Read the model definition and answer for the solid it produces. Units are mm, in the model's axes. A direction names the side the tool comes from. Coordinates: 2 decimals unless noted, no trailing zeros. Loops run counter-clockwise (first coordinate to the right, second up) from the corner with the lowest first, then second, coordinate; pieces in that order, holes last. Notation, with made-up numbers: (64, -11) - (98, -11) arc R28 cw to (98, 21) - close; hole circle Ø8 at (41.5, 37.5). An arc over 180 degrees is marked (long way). Use one line per item in the form item = value.
from build123d import *

# Parameters (mm, degrees)
F0_W      = 100
F0_H      = 100
F1_DEPTH  = 100
F2_R      = 5
F3_DEPTH  = 100
F5_DEPTH  = 25
F8_DEPTH  = 25
F10_DEPTH = 25
F11_DEPTH = 25
F12_SIZE  = 5
F14_DEPTH = 10


with BuildPart() as f1:
    # F0 (on Top) → F1 (new body)
    with BuildSketch(Plane.XY):
        with Locations((50, 50)):
            Rectangle(F0_W, F0_H)
    extrude(amount=F1_DEPTH)

    # F2 (on face) → F3 (cut)
    with BuildSketch(Plane.XY.offset(100)):
        with Locations((15, 25)):
            Circle(F2_R)
        with Locations((15, 50)):
            Circle(F2_R)
        with Locations((15, 75)):
            Circle(F2_R)
    extrude(amount=-F3_DEPTH, mode=Mode.SUBTRACT)

    # F4 (on face) → F5 (cut)
    with BuildSketch(Plane.XZ):
        with BuildLine():
            Line((39.7404471785, 30), (50, 30))
            Line((50, 30), (100, 30))
            Line((100, 30), (100, 100))
            Line((100, 100), (29.7404471785, 100))
            Line((29.7404471785, 100), (29.7404471785, 40))
            ThreePointArc((29.7404471785, 40), (32.6693793666, 32.9289321881), (39.7404471785, 30))
        make_face()
    extrude(amount=-F5_DEPTH, mode=Mode.SUBTRACT)

    # F7 (on face) → F8 (cut)
    with BuildSketch(Plane(origin=(0, 100, 0), x_dir=(-1, 0, 0), z_dir=(0, 1, 0))):
        with BuildLine():
            Line((-100, 30), (-39.7373309731, 30))
            ThreePointArc((-39.7373309731, 30), (-32.6662631613, 32.9289321881), (-29.7373309731, 40))
            Line((-29.7373309731, 40), (-29.7373309731, 100))
            Line((-29.7373309731, 100), (-100, 100))
            Line((-100, 100), (-100, 30))
        make_face()
    extrude(amount=-F8_DEPTH, mode=Mode.SUBTRACT)

    # F9 (on face) → F10 (cut)
    with BuildSketch(Plane.XZ.offset(-25)):
        Polygon((100, 100), (29.7404471785, 100), (100, 30), align=None)
    extrude(amount=-F10_DEPTH, mode=Mode.SUBTRACT)

    # F11 (cut): a face of the model
    f11_faces = [f1.faces().sort_by_distance(p)[0] for p in [
        (76.5801490595, 50, 76.6666666667),
    ]]
    extrude(f11_faces, amount=-F11_DEPTH, mode=Mode.SUBTRACT)

    # F12
    f12_edges = [f1.edges().sort_by_distance(p)[0] for p in [
        (100, 0, 15),
        (100, 100, 15),
    ]]
    chamfer(f12_edges, length=F12_SIZE)

    # F13 (on face) → F14 (cut)
    with BuildSketch(Plane.YZ.offset(100)):
        Polygon((39.8671727255, 10), (49.8671727255, 10), (59.8671727255, 10), (59.8671727255, 20.3688494319), (39.8671727255, 20.3688494319), align=None)
    extrude(amount=-F14_DEPTH, mode=Mode.SUBTRACT)


solid = f1.part
Item 1: The part is cut by section B-B on y = 50. Give the vertices of the cut face in (x, z), plus the area to 3 significant figures.
Results below:
outline = (0, 0) - (10, 0) - (10, 100) - (0, 100) - close; (20, 0) - (100, 0) - (100, 10) - (90, 10) - (90, 20.37) - (100, 20.37) - (100, 30) - (29.74, 100) - (20, 100) - close
area = 6,440 mm²
Item 2: Each of these flat-tipped pins is pushed along its axis until it touches: P1, Ø7.5, axis at y = 13.5, z = 69.5, coming from the +X side; P2, Ø20, axis at x = 56, y = 89, coming from the +Z side; P3, Ø3, axis at x = 97, z = 15.5, coming from the +Y side; P4, Ø6, axis at x = 15, y = 25, coming from the -Z side. Where does it stop, or does it pass through?
Results below:
P1 = 29.74
P2 = 30
P3 = 99.5
P4 = through
Item 3: The part is cut by section A-A on x = 15. Give the vertices of the cut face in (y, z).
Results below:
outline = (0, 0) - (20, 0) - (20, 100) - (0, 100) - close; (30, 0) - (45, 0) - (45, 100) - (30, 100) - close; (55, 0) - (70, 0) - (70, 100) - (55, 100) - close; (80, 0) - (100, 0) - (100, 100) - (80, 100) - close
Item 4: The part is cut by section C-C on z = 8.5. Give the vertices of the cut face in (x, y), plus the area to 3 significant figures.
Results below:
outline = (0, 0) - (95, 0) - (100, 5) - (100, 95) - (95, 100) - (0, 100) - close; hole circle Ø10 at (15, 25); hole circle Ø10 at (15, 50); hole circle Ø10 at (15, 75)
area = 9,740 mm²
Item 5: Which of the six approach directions +Z, -Z, +X, -X, +Y, -Y give full straight-line access (tool end or side, diameter ignored) to faces 4 (the flat face through (69, 12, 30)), 5 (the flat face through (97, 2, 15)), 6 (the flat face through (95, 50, 20.369)), 7 (the flat face through (29.737, 88, 70))?
Results below:
face_4 = +Z, +X, -Y
face_5 = +Z, -Z, +X, -Y
face_6 = +X
face_7 = +Z, +X, +Y
Item 6: The part is cut by section D-D on y = 86. Give the vertices of the cut face in (x, z), plus the area to 3 significant figures.
Results below:
outline = (0, 0) - (100, 0) - (100, 30) - (39.74, 30) arc R10 cw to (29.74, 40) - (29.74, 100) - (0, 100) - close
area = 5,100 mm²
Item 7: Find the intervals of material crossed by L1, parallel to Y at x = 15, z = 51.5; L2, parallel to Y at x = 11, z = 38.5; L3, parallel to Z at x = 47, y = 10, in increasing order.
Results below:
L1 = 0 to 20, 30 to 45, 55 to 70, 80 to 100
L2 = 0 to 22, 28 to 47, 53 to 72, 78 to 100
L3 = 0 to 30
Item 8: For a pull along X with two mould halves and no side action, classify faces 1 (the cylindrical face through (17.307, 20.564, 50.7)), 2 (the cylindrical face through (32.744, 87.675, 32.852)), 3 (the flat face through (26, 0, 38)) as +X half, -X half, draft (parallel to the pull), parting line (faces both ways), or undercut.
Results below:
face_1 = undercut
face_2 = +X half
face_3 = draft
